from build123d import *

# Parameters (mm, degrees)
SKETCH1_W           = 259
SKETCH1_H           = 175
BOSS_EXTRUDE1_DEPTH = 181
SKETCH2_R           = 9
SKETCH2_R_2         = 8
BOSS_EXTRUDE2_DEPTH = 22
SKETCH3_W           = 2.5
SKETCH3_H           = 3
SKETCH3_W_2         = 3
SKETCH3_H_2         = 2.5
SKETCH3_W_3         = 8
CUT_EXTRUDE1_DEPTH  = 1


with BuildPart() as part:
    # Sketch1 → Boss-Extrude1 (new body)
    with BuildSketch(Plane(origin=(0, 0, 0), x_dir=(1, 0, 0), z_dir=(0, 1, 0))):
        Rectangle(SKETCH1_W, SKETCH1_H)
    extrude(amount=BOSS_EXTRUDE1_DEPTH)

    # Sketch2 → Boss-Extrude2 (add)
    with BuildSketch(Plane(origin=(0, 181, 0), x_dir=(1, 0, 0), z_dir=(0, 1, 0))):
        with Locations(Location((-104.5, -47.5, 0), (0, 0, 270))):
            Circle(SKETCH2_R)
        with Locations(Location((104.5, -47.5, 0), (0, 0, 270))):
            Circle(SKETCH2_R_2)
    extrude(amount=BOSS_EXTRUDE2_DEPTH)

    # Sketch3 → Cut-Extrude1 (cut)
    with BuildSketch(Plane(origin=(0, 181, 0), x_dir=(1, 0, 0), z_dir=(0, 1, 0))):
        with Locations((-107.25, -72.5)):
            Rectangle(SKETCH3_W, SKETCH3_H)
        with Locations((-104.5, -72.5)):
            Rectangle(SKETCH3_W_2, SKETCH3_H)
        with Locations((-104.5, -69.75)):
            Rectangle(SKETCH3_W_2, SKETCH3_H_2)
        with Locations((-101.75, -72.5)):
            Rectangle(SKETCH3_W, SKETCH3_H)
        with Locations((-104.5, -75.25)):
            Rectangle(SKETCH3_W_2, SKETCH3_H_2)
        with Locations((104.5, -72.5)):
            Rectangle(SKETCH3_W_3, SKETCH3_H)
    extrude(amount=-CUT_EXTRUDE1_DEPTH, mode=Mode.SUBTRACT)


solid = part.part
Read the model definition and answer for the solid it produces. Units are mm, in the model's axes. A direction names the side the tool comes from. Round coordinates to 2 decimals unless told otherwise and drop trailing zeros. Loops run counter-clockwise (first coordinate to the right, second up) from the corner with the lowest first, then second, coordinate; pieces in that order, holes last. Notation, with made-up numbers: (31, -17.5) - (62, -17.5) arc R16 cw to (62, 8.5) - close; hole circle Ø3 at (-37.5, 84). An arc over 180 degrees is marked (long way). One line per question, with ' | ' between items. Start each with the question number.
Q1. For a pull along X with two mould halves and no side action, classify faces 3 (the flat face through (-2, 89, 87.5)), 4 (the flat face through (-105, 180, 72)), 5 (the flat face through (129.5, 89, 1)), 6 (the flat face through (-129.5, 89, 1)) as +X half, -X half, draft (parallel to the pull), parting line (faces both ways), or undercut.
Q2. For faces 1 (the cylindrical face through (-113.286, 191.846, 45.549)), 2 (the flat face through (105, 203, 47)), determine the directions among +Z, -Z, +X, -X, +Y, -Y from which every point of the face is accessible in a straight line to the end or side of a thin tool.
Q3. Section D-D on x = 28 is taken. Give the vertices of the cut face in (y, z).
Q4. Find the intervals of material crossed by L1, parallel to Y at x = -29, z = -76.5, in increasing order.
Q5. Section C-C on y = 185 is taken. Give the vertices of the cut face in (x, z), plus the area to 3 significant figures.
Q6. Flat-ended cylindrical pins translate along their axes: pin 1 (1 mm diameter, centred on x = 50, z = -25, fed in from +Y); pin 2 (0.9 mm diameter, centred on x = 106, z = 72, fed in from +Y); pin 3 (1.5 mm diameter, centred on x = -6, z = -11.5, fed in from -Y). Find the tip coordinate at first contact, or state that the pin passes through.
Q7. Section A-A on x = 104.5 is taken. Give the vertices of the cut face in (y, z), plus the area to 3 significant figures.
Q8. Section B-B on z = 47.5 is taken. Give the vertices of the cut face in (x, y), plus the area to 3 significant figures.
Established:
1) face 3: draft | face 4: undercut | face 5: +X half | face 6: -X half
2) face 1: +Y | face 2: +Z, -Z, +X, -X, +Y
3) outline: (0, -87.5) - (181, -87.5) - (181, 87.5) - (0, 87.5) - close
4) L1: 0 to 181
5) outline: circle Ø18 at (-104.5, 47.5); circle Ø16 at (104.5, 47.5) | area: 456 mm²
6) pin 1: y = 181 | pin 2: y = 180 | pin 3: y = 0
7) outline: (0, -87.5) - (181, -87.5) - (181, 39.5) - (203, 39.5) - (203, 55.5) - (181, 55.5) - (181, 71) - (180, 71) - (180, 74) - (181, 74) - (181, 87.5) - (0, 87.5) - close | area: 32,000 mm²
8) outline: (-129.5, 0) - (129.5, 0) - (129.5, 181) - (112.5, 181) - (112.5, 203) - (96.5, 203) - (96.5, 181) - (-95.5, 181) - (-95.5, 203) - (-113.5, 203) - (-113.5, 181) - (-129.5, 181) - close | area: 47,600 mm²
